```python
from build123d import *

# Parameters (mm, degrees)
SKETCH_1_W          = 74
SKETCH_1_H          = 14.8
EXTRUDE_1_DEPTH     = 14.8
SKETCH_2_W          = 10.25
SKETCH_2_H          = 10.25
CUT_EXTRUDE_1_DEPTH = 65
SKETCH_3_R          = 3.9
EXTRUDE_2_DEPTH     = 15
SKETCH_4_R          = 3.9
EXTRUDE_3_DEPTH     = 13
CHAMFER_1_SIZE      = 5
SKETCH_8_R          = 1.45
CUT_EXTRUDE_4_DEPTH = 43.8
SKETCH_9_W          = 7.8
SKETCH_9_H          = 7.8
SKETCH_9_R          = 1.5
EXTRUDE_4_DEPTH     = 3.55
SKETCH_10_W         = 7.8
SKETCH_10_H         = 7.8
EXTRUDE_5_DEPTH     = 3.55
SKETCH1_R           = 1.6
CUT_EXTRUDE1_DEPTH  = 30.8
SKETCH2_R           = 1.5
CUT_EXTRUDE2_DEPTH  = 43.8
SKETCH3_W           = 10.25
SKETCH3_H           = 3
CUT_EXTRUDE3_DEPTH  = 10


with BuildPart() as part:
    # Эскиз1 → Бобышка-Вытянуть1 (new body)
    with BuildSketch(Plane(origin=(0, 0, 0), x_dir=(0, 0, -1), z_dir=(1, 0, 0))):
        Rectangle(SKETCH_1_W, SKETCH_1_H)
    extrude(amount=EXTRUDE_1_DEPTH)

    # Эскиз2 → Вырез-Вытянуть1 (cut)
    with BuildSketch(Plane(origin=(0, 0, -37), x_dir=(-1, 0, 0), z_dir=(0, 0, -1))):
        with Locations((-7.4, 0)):
            Rectangle(SKETCH_2_W, SKETCH_2_H)
    extrude(amount=-CUT_EXTRUDE_1_DEPTH, mode=Mode.SUBTRACT)

    # Эскиз3 → Бобышка-Вытянуть2 (add)
    with BuildSketch(Plane(origin=(14.8, 0, 0), x_dir=(0, 0, -1), z_dir=(1, 0, 0))):
        with Locations((-33.1, 0)):
            Circle(SKETCH_3_R)
    extrude(amount=EXTRUDE_2_DEPTH)

    # Эскиз4 → Бобышка-Вытянуть3 (add)
    with BuildSketch(Plane.ZY):
        with Locations((33.1, 0)):
            Circle(SKETCH_4_R)
    extrude(amount=EXTRUDE_3_DEPTH)

    # Фаска1
    chamfer_1_edges = [part.edges().sort_by_distance(p)[0] for p in [
        (7.4, 7.4, 37),
        (7.4, -7.4, 37),
    ]]
    chamfer(chamfer_1_edges, length=CHAMFER_1_SIZE)

    # Эскиз8 → Вырез-Вытянуть4 (cut, through all)
    with BuildSketch(Plane(origin=(29.8, 0, 0), x_dir=(0, 0, -1), z_dir=(1, 0, 0))):
        with Locations((-33.1, 0)):
            Circle(SKETCH_8_R)
    extrude(amount=-CUT_EXTRUDE_4_DEPTH, mode=Mode.SUBTRACT)

    # Эскиз9 → Бобышка-Вытянуть4 (add)
    with BuildSketch(Plane.ZY):
        with Locations((33.1, 0)):
            Rectangle(SKETCH_9_W, SKETCH_9_H)
        with Locations((33.1, 0)):
            Circle(SKETCH_9_R, mode=Mode.SUBTRACT)
    extrude(amount=EXTRUDE_4_DEPTH)

    # Эскиз10 → Бобышка-Вытянуть5 (add)
    with BuildSketch(Plane(origin=(14.8, 0, 0), x_dir=(0, 0, -1), z_dir=(1, 0, 0))):
        with Locations((-33.1, 0)):
            Rectangle(SKETCH_10_W, SKETCH_10_H)
    extrude(amount=EXTRUDE_5_DEPTH)

    # Sketch1 → Cut-Extrude1 (cut, through all)
    with BuildSketch(Plane.ZY):
        with Locations((-33, -2.4)):
            Circle(SKETCH1_R)
    extrude(amount=-CUT_EXTRUDE1_DEPTH, mode=Mode.SUBTRACT)

    # Sketch2 → Cut-Extrude2 (cut, through all)
    with BuildSketch(Plane(origin=(29.8, 0, 0), x_dir=(0, 0, -1), z_dir=(1, 0, 0))):
        with Locations((-33.1, 0)):
            Circle(SKETCH2_R)
    extrude(amount=-CUT_EXTRUDE2_DEPTH, mode=Mode.SUBTRACT)

    # Sketch3 → Cut-Extrude3 (cut, through all)
    with BuildSketch(Plane(origin=(0, 0, 28), x_dir=(-1, 0, 0), z_dir=(0, 0, -1))):
        with Locations((-7.4, 3.625)):
            Rectangle(SKETCH3_W, SKETCH3_H)
    extrude(amount=-CUT_EXTRUDE3_DEPTH, mode=Mode.SUBTRACT)


solid = part.part
```
Design review of the part built by this model. Coordinates are the model's own, in mm. A direction names the side the tool comes from. Give positions to 0.01 mm unless a question says otherwise; leave off trailing zeros. Write each loop counter-clockwise with the first axis right and the second up, starting at its lowest first coordinate (ties: lowest second). Pieces come first, ordered by that corner, then holes. Notation, with made-up numbers: (20, 85) - (48, 85) arc R22 cw to (48, 116) - close; hole circle Ø1 at (-15, -16). An arc over 180 degrees is marked (long way). Return JSON: item names as keys, results as strings. Group by question number.
(1) To check wall thickness, follow probe 1 along X at (y, z) = (0, -15) (3 decimals); probe 2 along X at (y, z) = (-5.5, 23); probe 3 along Y at (x, z) = (14.2, -33). State the ranges of each line that lie inside material, in increasing order.
(2) Mouldability with a two-part tool opening along X and no side actions: class faces 5 (the flat face through (29.8, 0, 31)), 6 (the flat face through (-2, -3.9, 33)), 7 (the flat face through (2.275, 0, -1)) as +X half, -X half, draft (parallel to the pull), parting line (faces both ways), or undercut.
(3) We need section A-A, the plane x = 10. Give the boundary of the cut face in (y, z) (3 decimals).
(4) Machinability: for faces 1 (the flat face through (18.35, 3, 30)), 2 (the flat face through (-3.55, 3, 36)), 3 (the flat face through (12.525, 0, -1)), 4 (the flat face through (18.35, -3, 30)), which of the approach directions +Z, -Z, +X, -X, +Y, -Y give a long, thin tool a straight path to every point of the face, cutting with its end or side? Answer none if there is none.
(5) We need section C-C, the plane z = -33. Give the boundary of the cut face in (x, y) (3 decimals).
(6) We need section B-B, the plane z = -24. Give the boundary of the cut face in (x, y) (3 decimals).
(7) Insertion check: pin 1 (7.5 mm diameter, centred on y = -2, z = 9.5, fed in from -X); pin 2 (1.1 mm diameter, centred on x = 16, y = 0.5, fed in from -Z); pin 3 (1.8 mm diameter, centred on y = 0, z = 33.1, fed in from +X); pin 4 (4 mm diameter, centred on x = 16.5, z = 34, fed in from -Y). Each pin has a flat end and moves straight along its axis. Give the tip position at first contact, or say it passes through.
(8) We need section D-D, the plane x = 1. Give the boundary of the cut face in (y, z).
Reported:
{
 "1": {"probe 1": "x = 0 to 2.275, 12.525 to 14.8", "probe 2": "x = 0 to 14.8", "probe 3": "y = -7.4 to -4, -0.8 to 7.4"},
 "2": {"face 5": "+X half", "face 6": "draft", "face 7": "undercut"},
 "3": {"outline": "(-7.4, -37) - (-5.125, -37) - (-5.125, 28) - (2.125, 28) - (2.125, 37) - (-2.4, 37) - (-7.4, 32) - close; (5.125, -37) - (7.4, -37) - (7.4, 32) - (5.125, 34.275) - close; hole circle Ø3 at (0, 33.1)"},
 "4": {"face 1": "-Z, +X, +Y", "face 2": "+Z, -X, +Y", "face 3": "-Z", "face 4": "-Z, +X, -Y"},
 "5": {"outline": "(0, -7.4) - (14.8, -7.4) - (14.8, -4) - (12.525, -4) - (12.525, -5.125) - (2.275, -5.125) - (2.275, -4) - (0, -4) - close; (0, -0.8) - (2.275, -0.8) - (2.275, 5.125) - (12.525, 5.125) - (12.525, -0.8) - (14.8, -0.8) - (14.8, 7.4) - (0, 7.4) - close"},
 "6": {"outline": "(0, -7.4) - (14.8, -7.4) - (14.8, 7.4) - (0, 7.4) - close; hole (2.275, -5.125) - (12.525, -5.125) - (12.525, 5.125) - (2.275, 5.125) - close"},
 "7": {"pin 1": "stops at x = 0", "pin 2": "stops at z = 29.2", "pin 3": "passes through", "pin 4": "stops at y = -6.45"},
 "8": {"outline": "(-7.4, -37) - (7.4, -37) - (7.4, 32) - (2.4, 37) - (-2.4, 37) - (-7.4, 32) - close; hole circle Ø3.2 at (-2.4, -33); hole circle Ø3 at (0, 33.1)"}
}
